```python
from build123d import *

# Parameters (mm, degrees)
SKETCH_W        = 20
SKETCH_H        = 45
PAD_DEPTH       = 6
PAD001_DEPTH    = 15
SKETCH002_R     = 6
PAD002_DEPTH    = 6
SKETCH003_R     = 2
POCKET_DEPTH    = 6
SKETCH004_W     = 7
SKETCH004_H     = 6
POCKET001_DEPTH = 2
SKETCH005_W     = 16
SKETCH005_H     = 7
POCKET002_DEPTH = 2.5


with BuildPart() as part:
    # Sketch → Pad (new body)
    with BuildSketch(Plane.XY):
        with Locations((10, 22.5)):
            Rectangle(SKETCH_W, SKETCH_H)
    extrude(amount=PAD_DEPTH)

    # Sketch001 (on Face6 of Pad) → Pad001 (join)
    with BuildSketch(Plane.XY.offset(6)):
        Polygon((0, 0), (0, 45), (20, 45), (20, 41), (4, 41), (4, 0), align=None)
    extrude(amount=PAD001_DEPTH)

    # Sketch002 (on Face11 of Pad001) → Pad002 (join)
    with BuildSketch(Plane.XY.offset(21)):
        with BuildLine():
            Line((14, 0), (14, 41))
            Line((14, 41), (20, 41))
            Line((20, 41), (20, 57))
            ThreePointArc((20, 57), (5.683375, 67.488088), (0, 50.675445))
            Line((0, 50.675445), (0, 0))
            Line((14, 0), (0, 0))
        make_face()
        with Locations((9, 57)):
            Circle(SKETCH002_R, mode=Mode.SUBTRACT)
    extrude(amount=PAD002_DEPTH)

    # Sketch003 (on Face4 of Pad002) → Pocket (cut)
    with BuildSketch(Plane(origin=(0, 0, 0), x_dir=(1, 0, 0), z_dir=(0, 0, -1))):
        with Locations((9, -6)):
            Circle(SKETCH003_R)
        with Locations((9, -26)):
            Circle(SKETCH003_R)
        with Locations((15, -16)):
            Circle(SKETCH003_R)
    extrude(amount=-POCKET_DEPTH, mode=Mode.SUBTRACT)

    # Sketch004 (on Face20 of Pocket) → Pocket001 (cut)
    with BuildSketch(Plane.YZ.offset(14)):
        with Locations((37.5, 24)):
            Rectangle(SKETCH004_W, SKETCH004_H)
    extrude(amount=-POCKET001_DEPTH, mode=Mode.SUBTRACT)

    # Sketch005 (on Face6 of Pocket001) → Pocket002 (cut)
    with BuildSketch(Plane.XY.offset(6)):
        with Locations((12, 37.5)):
            Rectangle(SKETCH005_W, SKETCH005_H)
    extrude(amount=-POCKET002_DEPTH, mode=Mode.SUBTRACT)


solid = part.part
```
The model under review builds one solid part; all positions refer to its coordinate system, in mm. A direction names the side the tool comes from. Coordinates: 2 decimals unless noted, no trailing zeros. Write each loop counter-clockwise with the first axis right and the second up, starting at its lowest first coordinate (ties: lowest second). Pieces come first, ordered by that corner, then holes. Notation, with made-up numbers: (78.5, -19.5) -> (130.5, -19.5) arc R19 cw to (130.5, 13.5) -> close; hole circle Ø1 at (-4.5, -2.5). An arc over 180 degrees is marked (long way). One line per item, written item: value. Start each with the question number.
Q1. For faces 5 (the face through (12, 17, 6)), 6 (the face through (12, 34, 5)), 7 (the face through (7.4, 7.2, 3)), list the 3-axis set-ups (+Z, -Z, +X, -X, +Y, -Y) from which the entire face can be reached by the end or side of a thin tool; tool diameter is ignored.
Q2. To check wall thickness, follow probe 1 along Y at (x, z) = (9, 22.7); probe 2 along Z at (x, y) = (10.75, 13); probe 3 along X at (y, z) = (6, 2.45). State the ranges of each line that lie inside material, in increasing order.
Q3. Add section C-C, the plane x = 16. Give the boundary of the cut face in (y, z), then the cut area to 3 significant figures.
Q4. Clearance check with flat-ended pins moving along their axes: P1, Ø6, axis at x = 17, z = 6.5, coming from the -Y side; P2, Ø3, axis at y = 21, z = 23, coming from the +X side; P3, Ø12, axis at y = 29.5, z = 12.5, coming from the -X side; P4, Ø2, axis at x = 13.5, z = 23, coming from the +Y side. State where each tip first meets the part, or that it passes through.
Q5. The part is to be moulded in two halves that separate along X. For faces 1 (the face through (20, 30, 5)), 2 (the face through (12, 38, 3.5)), 3 (the face through (15, 14, 3)), 4 (the face through (3, 57, 24)), say which applies: +X half, -X half, draft (parallel to the pull), parting line (faces both ways), or undercut.
Q6. Add section D-D, the plane y = 35. Give the boundary of the cut face in (x, z), then the cut area to 3 significant figures.
Q7. Add section B-B, the plane z = 22. Give the boundary of the cut face in (x, y).
Q8. Add section A-A, the plane y = 26. Give the boundary of the cut face in (x, z).
Response:
1. face 5: +X, -Y
1. face 6: +X
1. face 7: -Z
2. probe 1: 0 to 51, 63 to 68
2. probe 2: 0 to 6, 21 to 27
2. probe 3: 0 to 7, 11 to 20
3. outline: (0, 0) -> (14.27, 0) -> (14.27, 6) -> (0, 6) -> close; (17.73, 0) -> (45, 0) -> (45, 21) -> (65.49, 21) -> (65.49, 27) -> (41, 27) -> (41, 3.5) -> (34, 3.5) -> (34, 6) -> (17.73, 6) -> close
3. area: 439 mm²
4. P1: y = 0
4. P2: x = 14
4. P3: x = 0
4. P4: y = 67.43
5. face 1: +X half
5. face 2: draft
5. face 3: undercut
5. face 4: undercut
6. outline: (0, 0) -> (20, 0) -> (20, 3.5) -> (4, 3.5) -> (4, 21) -> (12, 21) -> (12, 27) -> (0, 27) -> close
6. area: 212 mm²
7. outline: (0, 0) -> (14, 0) -> (14, 34) -> (12, 34) -> (12, 41) -> (20, 41) -> (20, 57) arc R11 ccw (long way) to (0, 50.68) -> close; hole circle Ø12 at (9, 57)
8. outline: (0, 0) -> (7, 0) -> (7, 6) -> (4, 6) -> (4, 21) -> (14, 21) -> (14, 27) -> (0, 27) -> close; (11, 0) -> (20, 0) -> (20, 6) -> (11, 6) -> close
